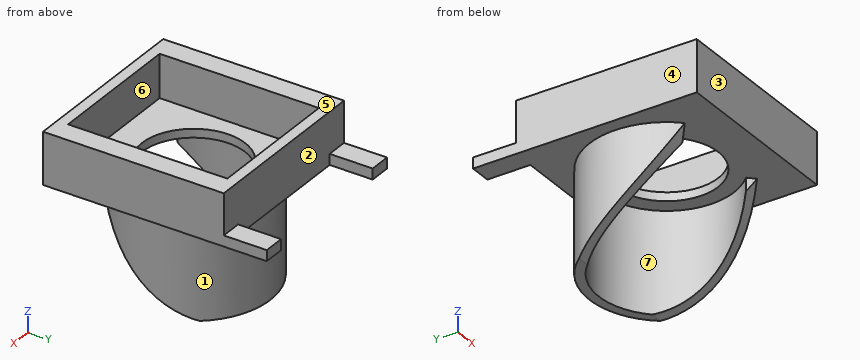
```python
from build123d import *

# Parameters (mm, degrees)
SKETCH2_W            = 350
SKETCH2_H            = 1050
SKETCH2_R            = 100
BOSS_EXTRUDE2_DEPTH  = 100
SCALE1_SCALE         = 0.24
SKETCH6_W            = 84
SKETCH6_H            = 168
CUT_EXTRUDE3_DEPTH   = 80
SKETCH11_W           = 64
SKETCH11_H           = 74
CUT_EXTRUDE8_DEPTH   = 20
SKETCH12_W           = 10
SKETCH12_H           = 5
BOSS_EXTRUDE6_DEPTH  = 20
SKETCH13_W           = 10
SKETCH13_H           = 5
BOSS_EXTRUDE7_DEPTH  = 20
SKETCH14_W           = 10
SKETCH14_H           = 5
CUT_EXTRUDE9_DEPTH   = 40
SKETCH15_W           = 10
SKETCH15_H           = 5
CUT_EXTRUDE10_DEPTH  = 40
SKETCH16_W           = 10
SKETCH16_H           = 20
CUT_EXTRUDE11_DEPTH  = 5
SKETCH17_W           = 10
SKETCH17_H           = 20
CUT_EXTRUDE12_DEPTH  = 5
BOSS_EXTRUDE9_DEPTH  = 47
SWEEP3_START         = -9
SWEEP3_DEPTH         = 47
CUT_EXTRUDE13_DEPTH  = 82
SKETCH28_W           = 10
SKETCH28_H           = 20
BOSS_EXTRUDE10_DEPTH = 5
SKETCH29_W           = 10
SKETCH29_H           = 20
BOSS_EXTRUDE11_DEPTH = 5
SKETCH30_W           = 10
SKETCH30_H           = 5
BOSS_EXTRUDE12_DEPTH = 40
SKETCH31_W           = 10
SKETCH31_H           = 5
BOSS_EXTRUDE13_DEPTH = 40


# Read off the part's stored shape, not the designer's step: Sweep3
with BuildPart() as part:
    # Sketch2 → Boss-Extrude2 (new body)
    with BuildSketch(Plane.XY):
        with Locations((13.505164405, -303.545290931)):
            Rectangle(SKETCH2_W, SKETCH2_H)
        with Locations((13.505164405, 46.454709069)):
            Circle(SKETCH2_R, mode=Mode.SUBTRACT)
        with Locations((13.505164405, -303.545290931)):
            Circle(SKETCH2_R, mode=Mode.SUBTRACT)
        with Locations((13.505164405, -653.545290931)):
            Circle(SKETCH2_R, mode=Mode.SUBTRACT)
    extrude(amount=BOSS_EXTRUDE2_DEPTH)


with BuildPart() as part_1:
    # Scale1: scaled about (13.505164405, -303.545290931, 50)
    add(part.part.scale(SCALE1_SCALE).moved(Location((10.263924948, -230.694421108, 38))))

    # Sketch6 → Cut-Extrude3 (cut)
    with BuildSketch(Plane.XY.offset(62)):
        with Locations((13.505164405, -261.545290931)):
            Rectangle(SKETCH6_W, SKETCH6_H)
    extrude(amount=-CUT_EXTRUDE3_DEPTH, mode=Mode.SUBTRACT)

    # Sketch11 → Cut-Extrude8 (cut)
    with BuildSketch(Plane.XY.offset(62)):
        with Locations((13.505164405, -387.545290931)):
            Rectangle(SKETCH11_W, SKETCH11_H)
    extrude(amount=-CUT_EXTRUDE8_DEPTH, mode=Mode.SUBTRACT)

    # Sketch12 → Boss-Extrude6 (add)
    with BuildSketch(Plane(origin=(0, -429.545290931, 0), x_dir=(-1, 0, 0), z_dir=(0, -1, 0))):
        with Locations((23.494835595, -40.5)):
            Rectangle(SKETCH12_W, SKETCH12_H)
    extrude(amount=BOSS_EXTRUDE6_DEPTH)

    # Sketch13 → Boss-Extrude7 (add)
    with BuildSketch(Plane(origin=(0, -429.545290931, 0), x_dir=(-1, 0, 0), z_dir=(0, -1, 0))):
        with Locations((-50.505164405, -40.5)):
            Rectangle(SKETCH13_W, SKETCH13_H)
    extrude(amount=BOSS_EXTRUDE7_DEPTH)

    # Sketch14 → Cut-Extrude9 (cut)
    with BuildSketch(Plane.XZ.offset(449.545290931)):
        with Locations((-23.494835595, 40.5)):
            Rectangle(SKETCH14_W, SKETCH14_H)
    extrude(amount=-CUT_EXTRUDE9_DEPTH, mode=Mode.SUBTRACT)

    # Sketch15 → Cut-Extrude10 (cut)
    with BuildSketch(Plane(origin=(0, -449.545290931, 0), x_dir=(-1, 0, 0), z_dir=(0, -1, 0))):
        with Locations((-50.505164405, -40.5)):
            Rectangle(SKETCH15_W, SKETCH15_H)
    extrude(amount=-CUT_EXTRUDE10_DEPTH, mode=Mode.SUBTRACT)

    # Sketch16 → Cut-Extrude11 (cut)
    with BuildSketch(Plane(origin=(0, 0, 38), x_dir=(-1, 0, 0), z_dir=(0, 0, -1))):
        with Locations((23.494835595, -355.545290931)):
            Rectangle(SKETCH16_W, SKETCH16_H)
    extrude(amount=-CUT_EXTRUDE11_DEPTH, mode=Mode.SUBTRACT)

    # Sketch17 → Cut-Extrude12 (cut)
    with BuildSketch(Plane(origin=(0, 0, 38), x_dir=(-1, 0, 0), z_dir=(0, 0, -1))):
        with Locations((-50.505164405, -355.545290931)):
            Rectangle(SKETCH17_W, SKETCH17_H)
    extrude(amount=-CUT_EXTRUDE12_DEPTH, mode=Mode.SUBTRACT)

    # Sketch18 → Boss-Extrude9 (add)
    with BuildSketch(Plane(origin=(0, 0, 38), x_dir=(-1, 0, 0), z_dir=(0, 0, -1))):
        with BuildLine():
            Line((-35.671185106, -409.711311632), (-38.7770157, -412.817142227))
            ThreePointArc((-38.7770157, -412.817142227), (-13.505164405, -351.805496082), (11.766686891, -412.817142227))
            Line((11.766686891, -412.817142227), (8.660856297, -409.711311632))
            ThreePointArc((8.660856297, -409.711311632), (-13.505164405, -356.197803831), (-35.671185106, -409.711311632))
        make_face()
    extrude(amount=BOSS_EXTRUDE9_DEPTH)


with BuildPart() as body_2:
    # Sweep3 outline → Sweep3 (new body)
    with BuildSketch(Plane.XY.offset(SWEEP3_START)):
        with BuildLine():
            Line((35.671185106, -409.711311632), (38.7770157, -412.817142227))
            ThreePointArc((38.7770157, -412.817142227), (13.505164405, -351.805496082), (-11.766686891, -412.817142227))
            Line((-11.766686891, -412.817142227), (-8.660856297, -409.711311632))
            ThreePointArc((-8.660856297, -409.711311632), (13.505164404, -356.197803831), (35.671185106, -409.711311632))
        make_face()
    extrude(amount=SWEEP3_DEPTH)


with BuildPart() as cut_extrude13_tool:
    # Sketch27 → Cut-Extrude13 (new body)
    with BuildSketch(Plane.ZY.offset(28.494835595)):
        with BuildLine():
            Line((38, -412.817142227), (-9, -412.817142227))
            Line((-9, -412.817142227), (-9, -365.817142227))
            add(Edge.make_bspline(
                [(-9, -365.817142227), (5.370162337, -397.723377267), (38, -412.817142227)],
                knots=[0, 0, 0, 1, 1, 1], degree=2))
        make_face()
    extrude(amount=-CUT_EXTRUDE13_DEPTH)


with BuildPart() as part_2:
    add(part_1.part)

    # Cut-Extrude13: cut by cut_extrude13_tool
    add(cut_extrude13_tool.part, mode=Mode.SUBTRACT)



with BuildPart() as body_2_1:
    add(body_2.part)

    # Cut-Extrude13: cut by cut_extrude13_tool
    add(cut_extrude13_tool.part, mode=Mode.SUBTRACT)


with BuildPart() as part_3:
    add(part_2.part)

    add(body_2_1.part)  # Boss-Extrude10 merges body 2
    # Sketch28 → Boss-Extrude10 (add)
    with BuildSketch(Plane(origin=(0, 0, 43), x_dir=(-1, 0, 0), z_dir=(0, 0, -1))):
        with Locations((-50.505164405, -419.545290931)):
            Rectangle(SKETCH28_W, SKETCH28_H)
    extrude(amount=BOSS_EXTRUDE10_DEPTH)

    # Sketch29 → Boss-Extrude11 (add)
    with BuildSketch(Plane(origin=(0, 0, 43), x_dir=(-1, 0, 0), z_dir=(0, 0, -1))):
        with Locations((23.494835595, -419.545290931)):
            Rectangle(SKETCH29_W, SKETCH29_H)
    extrude(amount=BOSS_EXTRUDE11_DEPTH)

    # Sketch30 → Boss-Extrude12 (add)
    with BuildSketch(Plane(origin=(0, -365.545290931, 0), x_dir=(1, 0, 0), z_dir=(0, 1, 0))):
        with Locations((50.505164405, -40.5)):
            Rectangle(SKETCH30_W, SKETCH30_H)
    extrude(amount=BOSS_EXTRUDE12_DEPTH)

    # Sketch31 → Boss-Extrude13 (add)
    with BuildSketch(Plane(origin=(0, -365.545290931, 0), x_dir=(1, 0, 0), z_dir=(0, 1, 0))):
        with Locations((-23.494835595, -40.5)):
            Rectangle(SKETCH31_W, SKETCH31_H)
    extrude(amount=BOSS_EXTRUDE13_DEPTH)


solid = part_3.part
```
Design review of the part built by this model. Coordinates are the model's own, in mm. Face numbers are marked on the shaded views. A direction names the side the tool comes from. Round coordinates to 2 decimals unless told otherwise and drop trailing zeros. Order: outer loops, then holes, each group sorted by start corner. A loop starts at its lowest first (then second) coordinate and runs counter-clockwise, first axis right, second up. Notation, with made-up numbers: (20.25, 43) - (24.25, 43) arc R24 ccw to (24.25, 82) - close; hole circle Ø4 at (77.25, -2.5). An arc over 180 degrees is marked (long way). Return JSON: item names as keys, results as strings.
Q1. The part is to be moulded in two halves that separate along X. For the marked faces 1, 2, 3 and 4, say which applies: pulls with the +X half, pulls with the -X half, needs draft (parallel to the pull), parting line crosses it, or undercut.
Computed values:
{"face 1": "parting line crosses it", "face 2": "undercut", "face 3": "needs draft", "face 4": "pulls with the -X half"}
Q2. Wall thickness on L1, parallel to Y at x = 14, z = 48; L2, parallel to X at y = -362.5, z = 50.5; L3, parallel to Z at x = 18, y = -352.5: over which ranges is each line inside the solid? List them lowest first. Write a range as [from, to].
Computed values:
{"L1": "y = [-429.55, -424.55], [-350.55, -345.55]", "L2": "x = [-28.49, -18.49], [45.51, 55.51]", "L3": "z = [-9, 42]"}
Q3. Machinability: for the marked faces 5, 6 and 7, which of the approach directions +Z, -Z, +X, -X, +Y, -Y give a long, thin tool a straight path to every point of the face, cutting with its end or side? Answer none if there is none.
Computed values:
{"face 5": "+Z, +X, -X, +Y, -Y", "face 6": "+Z", "face 7": "-Z"}
Q4. Consider section C-C on z = 47.5. Write out the cut boundary in (x, y).
Computed values:
{"outline": "(-28.49, -429.55) - (55.51, -429.55) - (55.51, -345.55) - (-28.49, -345.55) - close; hole (-18.49, -424.55) - (45.51, -424.55) - (45.51, -350.55) - (-18.49, -350.55) - close"}
Q5. Consider section A-A on y = -339. Write out the cut boundary in (x, z), plus the area to 3 significant figures.
Computed values:
{"outline": "(-28.49, 38) - (-18.49, 38) - (-18.49, 43) - (-28.49, 43) - close; (45.51, 38) - (55.51, 38) - (55.51, 43) - (45.51, 43) - close", "area": "100 mm2"}
Q6. For pin 1 Ø3 at (x, y) = (6, -359) entering from -Z; pin 2 Ø6 at (x, z) = (26, 52) entering from +Y; pin 3 Ø3 at (x, y) = (-21, -331) entering from +Z; pin 4 Ø10 at (y, z) = (-354, 37.5) entering from +X, all flat-tipped, find the tip position at first contact; note any pin that passes through.
Computed values:
{"pin 1": "stops at z = 38", "pin 2": "stops at y = -345.55", "pin 3": "stops at z = 43", "pin 4": "stops at x = 55.51"}
Q7. Consider section D-D on y = -417.5. Write out the cut boundary in (x, z).
Computed values:
{"outline": "(-28.49, 38) - (55.51, 38) - (55.51, 62) - (45.51, 62) - (45.51, 42) - (-18.49, 42) - (-18.49, 62) - (-28.49, 62) - close"}
Q8. Consider section B-B on x = 1. Write out the cut boundary in (y, z), plus the area to 3 significant figures.
Computed values:
{"outline": "(-429.55, 38) - (-408.03, 38) - (-408.03, 42) - (-424.55, 42) - (-424.55, 62) - (-429.55, 62) - close; (-367.06, 38) - (-358.8, 38) - (-358.8, -9) - (-354.06, -9) - (-354.06, 38) - (-345.55, 38) - (-345.55, 62) - (-350.55, 62) - (-350.55, 42) - (-367.06, 42) - close", "area": "595 mm2"}
